```python
from build123d import *

# Parameters (mm, degrees)
SKETCH1_W           = 3.05
SKETCH1_H           = 10
SKETCH1_R           = 5
BOSS_EXTRUDE1_DEPTH = 3
CUT_EXTRUDE1_DEPTH  = 3
FILLET1_R           = 0.5


with BuildPart() as part:
    # Sketch1 → Boss-Extrude1 (new body)
    with BuildSketch(Plane(origin=(0, 0, 0), x_dir=(0, 0, -1), z_dir=(1, 0, 0))):
        with BuildLine():
            Line((-125, 13.75), (-125, -13.75))
            Line((-125, -13.75), (-109.166666667, -13.75))
            Line((-109.166666667, -13.75), (-109.166666667, -10.75))
            Line((-109.166666667, -10.75), (-93.333333333, -10.75))
            Line((-93.333333333, -10.75), (-93.333333333, -13.75))
            Line((-93.333333333, -13.75), (-77.5, -13.75))
            Line((-77.5, -13.75), (-77.5, -10.75))
            Line((-77.5, -10.75), (-61.666666667, -10.75))
            Line((-61.666666667, -10.75), (-61.666666667, -13.75))
            Line((-61.666666667, -13.75), (-45.833333333, -13.75))
            Line((-45.833333333, -13.75), (-45.833333333, -10.75))
            Line((-45.833333333, -10.75), (-30, -10.75))
            Line((-30, -10.75), (-30, -13.75))
            Line((-30, -13.75), (-14.166666667, -13.75))
            Line((-14.166666667, -13.75), (-14.166666667, -10.75))
            Line((-14.166666667, -10.75), (1.666666667, -10.75))
            Line((1.666666667, -10.75), (1.666666667, -13.75))
            Line((1.666666667, -13.75), (17.5, -13.75))
            Line((17.5, -13.75), (17.5, -10.75))
            Line((17.5, -10.75), (33.333333333, -10.75))
            Line((33.333333333, -10.75), (33.333333333, -13.75))
            Line((33.333333333, -13.75), (49.166666667, -13.75))
            Line((49.166666667, -13.75), (49.166666667, -10.75))
            Line((49.166666667, -10.75), (65, -10.75))
            Line((65, -10.75), (65, -13.75))
            Line((65, -13.75), (87.434301396, -13.75))
            ThreePointArc((87.434301396, -13.75), (138.75, 0), (87.434301396, 13.75))
            Line((87.434301396, 13.75), (65, 13.75))
            Line((65, 13.75), (65, 10.75))
            Line((65, 10.75), (49.166666667, 10.75))
            Line((49.166666667, 10.75), (49.166666667, 13.75))
            Line((49.166666667, 13.75), (33.333333333, 13.75))
            Line((33.333333333, 13.75), (33.333333333, 10.75))
            Line((33.333333333, 10.75), (17.5, 10.75))
            Line((17.5, 10.75), (17.5, 13.75))
            Line((17.5, 13.75), (1.666666667, 13.75))
            Line((1.666666667, 13.75), (1.666666667, 10.75))
            Line((1.666666667, 10.75), (-14.166666667, 10.75))
            Line((-14.166666667, 10.75), (-14.166666667, 13.75))
            Line((-14.166666667, 13.75), (-30, 13.75))
            Line((-30, 13.75), (-30, 10.75))
            Line((-30, 10.75), (-45.833333333, 10.75))
            Line((-45.833333333, 10.75), (-45.833333333, 13.75))
            Line((-45.833333333, 13.75), (-61.666666667, 13.75))
            Line((-61.666666667, 13.75), (-61.666666667, 10.75))
            Line((-61.666666667, 10.75), (-77.5, 10.75))
            Line((-77.5, 10.75), (-77.5, 13.75))
            Line((-77.5, 13.75), (-93.333333333, 13.75))
            Line((-93.333333333, 13.75), (-93.333333333, 10.75))
            Line((-93.333333333, 10.75), (-109.166666667, 10.75))
            Line((-109.166666667, 10.75), (-109.166666667, 13.75))
            Line((-109.166666667, 13.75), (-125, 13.75))
        make_face()
        Polygon((104.432289187, -6.789288937), (106.89979102, -8.582033956), (101.021938497, -16.6722039), (98.554436664, -14.879458881), align=None, mode=Mode.SUBTRACT)
        Polygon((115.60020898, -8.582033956), (118.067710813, -6.789288937), (123.945563336, -14.879458881), (121.478061503, -16.6722039), align=None, mode=Mode.SUBTRACT)
        Polygon((120.756287821, 1.485300259), (119.813785988, 4.386022634), (129.324351151, 7.476192578), (130.266852984, 4.575470203), align=None, mode=Mode.SUBTRACT)
        with Locations((111.25, 14.5)):
            Rectangle(SKETCH1_W, SKETCH1_H, mode=Mode.SUBTRACT)
        with Locations((-111.25, 0)):
            Circle(SKETCH1_R, mode=Mode.SUBTRACT)
        with Locations((111.25, 0)):
            Circle(SKETCH1_R, mode=Mode.SUBTRACT)
        Polygon((102.686214012, 4.386022634), (101.743712179, 1.485300259), (92.233147016, 4.575470203), (93.175648849, 7.476192578), align=None, mode=Mode.SUBTRACT)
    extrude(amount=BOSS_EXTRUDE1_DEPTH)

    # Sketch3 → Cut-Extrude1 (cut)
    with BuildSketch(Plane(origin=(3, 0, 0), x_dir=(0, 0, -1), z_dir=(1, 0, 0))):
        Polygon((-102.25, 0), (-102.25, -6.25), (-83.618433679, -6.25), align=None)
        Polygon((-54.004487489, 6.25), (-101.701297271, 6.25), (-77.85289238, -1.75), align=None)
        Polygon((-48.23894619, 1.75), (-72.087351081, -6.25), (-24.390541299, -6.25), align=None)
        Polygon((5.223404891, 6.25), (-42.473404891, 6.25), (-18.625, -1.75), align=None)
        Polygon((10.98894619, 1.75), (-12.859458701, -6.25), (34.837351081, -6.25), align=None)
        Polygon((64.451297271, 6.25), (16.754487489, 6.25), (40.60289238, -1.75), align=None)
        Polygon((65, 0), (46.368433679, -6.25), (65, -6.25), align=None)
    extrude(amount=-CUT_EXTRUDE1_DEPTH, mode=Mode.SUBTRACT)

    # Fillet1
    fillet1_edges = [part.edges().sort_by_distance(p)[0] for p in [
        (1.5, -1.75, 18.625),
        (1.5, 6.25, 42.473404891),
        (1.5, 6.25, -5.223404891),
        (1.5, 1.75, -10.98894619),
        (1.5, -6.25, -34.837351081),
        (1.5, -6.25, 12.859458701),
        (1.5, -1.75, 77.85289238),
        (1.5, 6.25, 101.701297271),
        (1.5, 6.25, 54.004487489),
        (1.5, 1.75, 48.23894619),
        (1.5, -6.25, 24.390541299),
        (1.5, -6.25, 72.087351081),
        (1.5, -6.25, -46.368433679),
        (1.5, 0, -65),
        (1.5, -6.25, -65),
        (1.5, -1.75, -40.60289238),
        (1.5, 6.25, -16.754487489),
        (1.5, 6.25, -64.451297271),
        (1.5, 0, 102.25),
        (1.5, -6.25, 83.618433679),
        (1.5, -6.25, 102.25),
    ]]
    fillet(fillet1_edges, radius=FILLET1_R)


solid = part.part
```
For this review, take the finished solid that the model builds, in its own axes (mm). A direction names the side the tool comes from. Round coordinates to 2 decimals unless told otherwise and drop trailing zeros. Write each loop counter-clockwise with the first axis right and the second up, starting at its lowest first coordinate (ties: lowest second). Pieces come first, ordered by that corner, then holes. Notation, with made-up numbers: (86, -9.75) - (115, -9.75) arc R15 cw to (115, -5.75) - close; hole circle Ø4 at (-1.5, 5). An arc over 180 degrees is marked (long way). Use CSV: the item, a comma, the result in double quotes.
1) Add section A-A on z = 84. Write out the cut boundary in (x, y), and give its area (3 significant figures).
Conclusion:
outline,"(0, -13.75) - (3, -13.75) - (3, 0.31) - (0, 0.31) - close; (0, 6.25) - (3, 6.25) - (3, 13.75) - (0, 13.75) - close"
area,"64.7 mm^2"
2) Add section B-B on x = 1.3. Count the separate pieces of the cut face and the enclosed holes in it, and give its area (3 significant figures).
Conclusion:
separate pieces,"1"
enclosed holes,"14"
area,"6,210 mm^2"
3) The part is to be moulded in two halves that separate along Z. For faces 3 (the flat face through (1.52, 1.74, 67.45)), 4 (the flat face through (0, 6.5, -34.3)), 5 (the flat face through (1.521, -1.741, 58.645)), say which applies: pulls with the +Z half, pulls with the -Z half, needs draft (parallel to the pull), parting line crosses it, or undercut.
Conclusion:
face 3,"undercut"
face 4,"needs draft"
face 5,"undercut"
4) For faces 1 (the flat face through (1.52, -1.74, -0.58)), 2 (the flat face through (3, 6.5, -34.3)), list the 3-axis set-ups (+Z, -Z, +X, -X, +Y, -Y) from which the entire face can be reached by the end or side of a thin tool; tool diameter is ignored.
Conclusion:
face 1,"+X, -X"
face 2,"+Z, -Z, +X, +Y, -Y"
5) Wall thickness on line 1 along Y through (x, z) = (0.9, 111.25); line 2 along Y through (x, z) = (1.95, -111.25); line 3 along Y through (x, z) = (1.2, -112): over which ranges is each line inside the solid? List them lowest first. Write a range as from..to.
Conclusion:
line 1,"y = -13.75..-5, 5..13.75"
line 2,"y = -27.5..-5, 5..9.5, 19.5..27.5"
line 3,"y = -27.49..-4.94, 4.94..9.5, 19.5..27.49"
6) Clearance check with flat-ended pins moving along their axes: pin 1 Ø1.5 at (x, z) = (1.5, 102.5) entering from +Y; pin 2 Ø1.5 at (x, z) = (2, 69) entering from -Y; pin 3 Ø10 at (y, z) = (19, 96.5) entering from -X; pin 4 Ø0.9 at (x, z) = (1.5, -78.5) entering from -Y. State where each tip first meets the part, or that it passes through.
Conclusion:
pin 1,"stops at y = 10.75"
pin 2,"stops at y = -10.75"
pin 3,"passes through"
pin 4,"stops at y = -13.75"
